```python
from build123d import *

# Parameters (mm, degrees)
SKETCH1_W           = 50
SKETCH1_H           = 20
SKETCH1_R           = 1.5
SKETCH1_R_2         = 2.35
SKETCH1_W_2         = 7.32
SKETCH1_H_2         = 3
SKETCH1_W_3         = 47
SKETCH1_H_3         = 2
BOSS_EXTRUDE1_DEPTH = 10


with BuildPart() as part:
    # Sketch1 → Boss-Extrude1 (new body)
    with BuildSketch(Plane.XY):
        with Locations((0, 2.450714286)):
            Rectangle(SKETCH1_W, SKETCH1_H)
        with Locations((-10, 7.450714286)):
            Circle(SKETCH1_R, mode=Mode.SUBTRACT)
        with Locations((10, 7.450714286)):
            Circle(SKETCH1_R, mode=Mode.SUBTRACT)
        with Locations((0, 7.450714286)):
            Circle(SKETCH1_R_2, mode=Mode.SUBTRACT)
        Rectangle(SKETCH1_W_2, SKETCH1_H_2, mode=Mode.SUBTRACT)
        with Locations((0, -4.5)):
            Rectangle(SKETCH1_W_3, SKETCH1_H_3, mode=Mode.SUBTRACT)
    extrude(amount=BOSS_EXTRUDE1_DEPTH)


solid = part.part
```
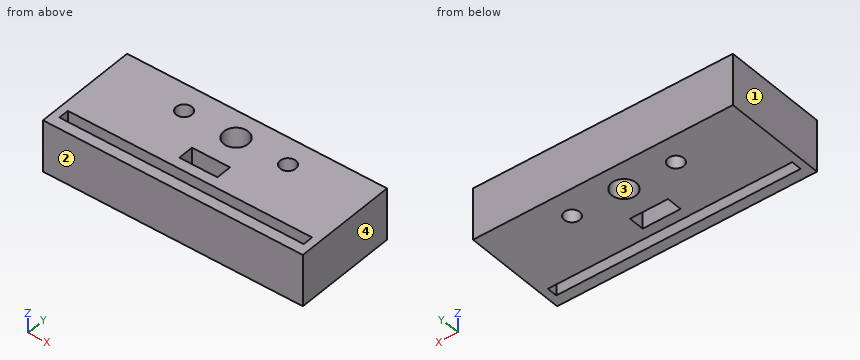
Here's how the part is built. I have some questions about the finished solid (model axes, mm). Face numbers are marked on the shaded views. Coordinates: 2 decimals unless noted, no trailing zeros. Order: outer loops, then holes, each group sorted by start corner. A loop starts at its lowest first (then second) coordinate and runs counter-clockwise, first axis right, second up.
Item 1: I need wall thicknesses on probe 1 along Y at (x, z) = (0, 5.75); probe 2 along Y at (x, z) = (10, 3.25); probe 3 along Y at (x, z) = (17, 5). Which ranges of each line are inside material? Lowest first, please.
Response values:
probe 1: y = -7.55 to -5.5, -3.5 to -1.5, 1.5 to 5.1, 9.8 to 12.45
probe 2: y = -7.55 to -5.5, -3.5 to 5.95, 8.95 to 12.45
probe 3: y = -7.55 to -5.5, -3.5 to 12.45
Item 2: If we section it at D-D, the plane x = -17: List the corners of the cut face in (y, z) for me, then the cut area to 3 significant figures.
Response values:
outline: (-7.55, 0) - (-5.5, 0) - (-5.5, 10) - (-7.55, 10) - close; (-3.5, 0) - (12.45, 0) - (12.45, 10) - (-3.5, 10) - close
area: 180 mm2
Item 3: If we section it at A-A, the plane y = 0.5: List the corners of the cut face in (x, z) for me, then the cut area to 3 significant figures.
Response values:
outline: (-25, 0) - (-3.66, 0) - (-3.66, 10) - (-25, 10) - close; (3.66, 0) - (25, 0) - (25, 10) - (3.66, 10) - close
area: 427 mm2
Item 4: If we section it at C-C, the plane x = 10: List the corners of the cut face in (y, z) for me.
Response values:
outline: (-7.55, 0) - (-5.5, 0) - (-5.5, 10) - (-7.55, 10) - close; (-3.5, 0) - (5.95, 0) - (5.95, 10) - (-3.5, 10) - close; (8.95, 0) - (12.45, 0) - (12.45, 10) - (8.95, 10) - close
Item 5: Thinking about a two-plate mould opening in X: for the marked faces 1, 2, 3 and 4, which applies, pulls with the +X half, pulls with the -X half, needs draft (parallel to the pull), parting line crosses it, or undercut?
Response values:
face 1: pulls with the -X half
face 2: needs draft
face 3: undercut
face 4: pulls with the +X half
Item 6: If we section it at B-B, the plane x = 0: List the corners of the cut face in (y, z) for me.
Response values:
outline: (-7.55, 0) - (-5.5, 0) - (-5.5, 10) - (-7.55, 10) - close; (-3.5, 0) - (-1.5, 0) - (-1.5, 10) - (-3.5, 10) - close; (1.5, 0) - (5.1, 0) - (5.1, 10) - (1.5, 10) - close; (9.8, 0) - (12.45, 0) - (12.45, 10) - (9.8, 10) - close
